Source: CAD feature listing. Evaluate the final solid. Frame: model axes, mm. Face numbers are marked on the shaded views. A direction names the side the tool comes from. Round coordinates to 2 decimals unless told otherwise and drop trailing zeros. Loops run counter-clockwise (first coordinate to the right, second up) from the corner with the lowest first, then second, coordinate; pieces in that order, holes last. Notation, with made-up numbers: M 81.25,61.5 L 105.25,61.5 A28 ccw 105.25,80.5 Z; hole C 6,87.5 d6. An arc over 180 degrees is marked long. Answer as a JSON object with one key per item and string values.
from build123d import *

# Parameters (mm, degrees)
SKETCH001_R     = 6
POCKET_DEPTH    = 8.820854
CHAMFER_SIZE    = 1
CHAMFER001_SIZE = 0.2


with BuildPart() as pocket:
    # Sketch003 → Revolution001 (revolve)
    with BuildSketch(Plane.XZ):
        Polygon((0, 1.180146), (5, 3), (5, 10), (0, 10), align=None)
    revolve(axis=Axis((0, 0, 0), (0, 0, 1)))

    # Sketch001 → Pocket (cut, through all)
    with BuildSketch(Plane(origin=(0, 0, 10), x_dir=(-1, 0, 0), z_dir=(0, 0, 1))):
        Circle(SKETCH001_R)
        Polygon((-1.443376, 2.5), (1.443376, 2.5), (2.886751, 0), (1.443376, -2.5), (-1.443376, -2.5), (-2.886751, 0), align=None, mode=Mode.SUBTRACT)
    extrude(amount=-POCKET_DEPTH, mode=Mode.SUBTRACT)


with BuildPart() as chamfer001:
    # Sketch → Revolution (revolve)
    with BuildSketch(Plane.XZ):
        Polygon((2.88675, 6), (5, 6), (5, 0), (3, 0), (3, -12), (0, -12), (0, 3.113247), align=None)
    revolve(axis=Axis((0, 0, 0), (0, 0, 1)))

    # Cut: cut Pocket
    add(pocket.part, mode=Mode.SUBTRACT)

    # Chamfer
    chamfer_edges = [chamfer001.edges().sort_by_distance(p)[0] for p in [
        (-3, 0, -12),
    ]]
    chamfer(chamfer_edges, length=CHAMFER_SIZE)

    # Chamfer001
    chamfer001_edges = [chamfer001.edges().sort_by_distance(p)[0] for p in [
        (-5, 0, 6),
        (-5, 0, 0),
    ]]
    chamfer(chamfer001_edges, length=CHAMFER001_SIZE)


solid = chamfer001.part
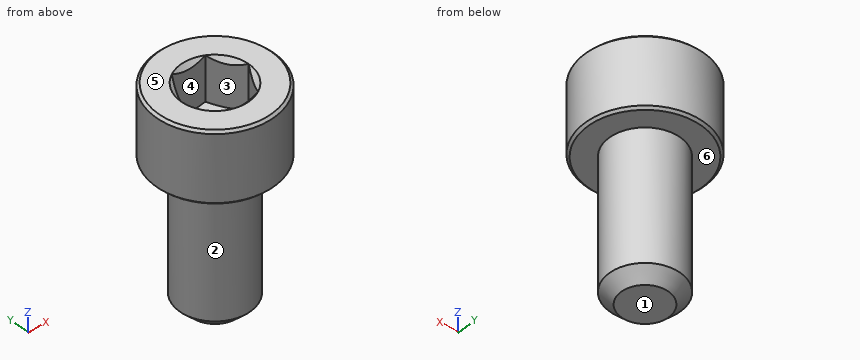
Item 1: Access query for the marked faces 4, 5 and 6. Directions: +Z, -Z, +X, -X, +Y, -Y. A direction counts if a zero-diameter tool reaches every point of the face in a straight line with its end or side. Return the directions, or none.
Answer sheet:
{"face 4": "+Z", "face 5": "+Z, +X, -X, +Y, -Y", "face 6": "-Z"}
Item 2: Contact query for flat-ended pins moving along their axis: pin 1 Ø4 at (y, z) = (-2, 1) entering from -X; pin 2 Ø2 at (y, z) = (-3, -0.5) entering from -X; pin 3 Ø5 at (x, z) = (-2.5, -10) entering from +Y; pin 4 Ø2 at (x, z) = (3, -9) entering from -Y. Output: stop coordinate, or through.
Answer sheet:
{"pin 1": "stops at x = -5", "pin 2": "stops at x = -4.45", "pin 3": "stops at y = 3", "pin 4": "stops at y = -2.24"}
Item 3: Section B-B on z = -9.25. Return the cut outline in (x, y).
Answer sheet:
{"outline": "C 0,0 d6"}
Item 4: Pull-direction query (X, two-part tool) for the marked faces 1, 2 and 3; classes: pulls with the +X half, pulls with the -X half, needs draft (parallel to the pull), parting line crosses it, or undercut.
Answer sheet:
{"face 1": "needs draft", "face 2": "parting line crosses it", "face 3": "undercut"}
Item 5: Section A-A on z = 3. Return the cut outline in (x, y).
Answer sheet:
{"outline": "C 0,0 d10; hole M -2.89,0 L -1.44,-2.5 L 1.44,-2.5 L 2.89,0 L 1.44,2.5 L -1.44,2.5 Z"}
Item 6: Line query: probe 1 along Z at (x, y) = (0, 0); probe 2 along Y at (x, z) = (0.25, 2.25); probe 3 along X at (y, z) = (-4, 0.5). Output: solid intervals per line, ascending. Write a range as from..to.
Answer sheet:
{"probe 1": "z = -12..1.18", "probe 2": "y = -4.99..-2.5, 2.5..4.99", "probe 3": "x = -3..3"}
